Verification items for this drawing (mm, ordinates from the low corner). A direction names the side the tool comes from. Coordinates: 2 decimals unless noted, no trailing zeros. Order: outer loops, then holes, each group sorted by start corner. A loop starts at its lowest first (then second) coordinate and runs counter-clockwise, first axis right, second up. Notation, with made-up numbers: (33, -17) -> (70, -17) arc R22 cw to (70, 8) -> close; hole circle Ø11 at (61.5, 20.5). An arc over 180 degrees is marked (long way). Write item = value, one per line. Start each with the question number.
1. Cross-section at C-C on z = 12.7. Record the cut outline in (x, y).
2. Set-up check for the marked faces 4, 5, 6 and 7: record each of +Z, -Z, +X, -X, +Y, -Y from which the full face is reachable in a straight line by a thin tool's end or side.
3. Thickness scan on line 1 along Z through (x, y) = (18, 38.1); line 2 along Y through (x, z) = (19, 38.5); line 3 along Y through (x, z) = (23.5, 28.5). Record the ranges inside material, lowest first. Write a range as from..to.
4. Cross-section at A-A on y = 38.1. Record the cut outline in (x, z), plus the area to 3 significant figures.
5. Go/stop test with flat-tipped pins: P1, Ø12.5, axis at x = 11, y = 41, coming from the -Z side; P2, Ø12, axis at y = 8.5, z = 22, coming from the -X side; P3, Ø1, axis at x = 10, z = 43.5, coming from the -Y side. Record where each tip stops, or that it passes through.
6. Cross-section at D-D on x = 38.1. Record the cut outline in (y, z), plus the area to 3 significant figures.
7. Release check for a two-part mould opening along X. For the marked faces 1, 2 and 3 record: +X half, -X half, draft (parallel to the pull), parting line (faces both ways), or undercut.
8. Cross-section at B-B on x = 21. Record the cut outline in (y, z).
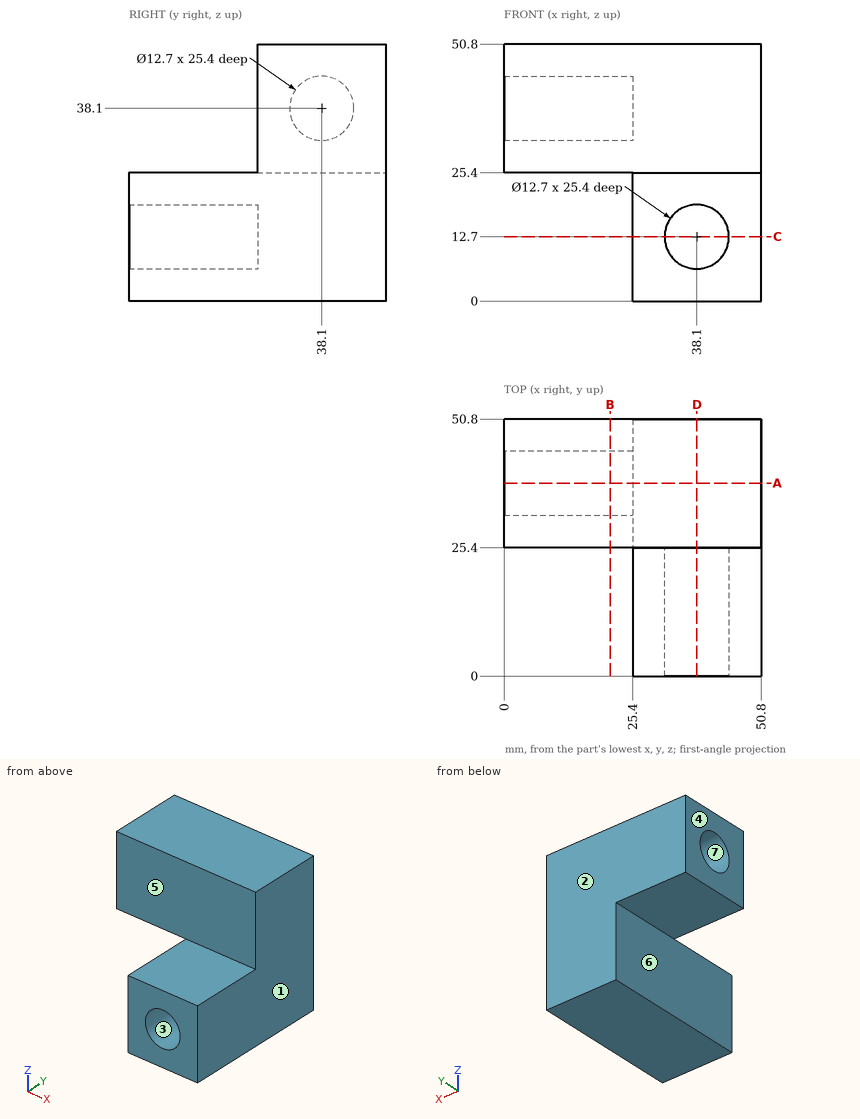
Worked out:
q1.outline = (25.4, 0) -> (31.75, 0) -> (31.75, 25.4) -> (44.45, 25.4) -> (44.45, 0) -> (50.8, 0) -> (50.8, 50.8) -> (25.4, 50.8) -> close
q2.face_4 = +Z, -Z, -X, +Y, -Y
q2.face_5 = +Z, +X, -X, -Y
q2.face_6 = -Z, -X, +Y, -Y
q2.face_7 = -X
q3.line_1 = 25.4..31.75, 44.45..50.8
q3.line_2 = 25.4..31.76, 44.44..50.8
q3.line_3 = 25.4..50.8
q4.outline = (0, 25.4) -> (25.4, 25.4) -> (25.4, 0) -> (50.8, 0) -> (50.8, 50.8) -> (0, 50.8) -> (0, 44.45) -> (25.4, 44.45) -> (25.4, 31.75) -> (0, 31.75) -> close
q4.area = 1,610 mm²
q5.P1 = 25.4
q5.P2 = 25.4
q5.P3 = 25.4
q6.outline = (0, 0) -> (50.8, 0) -> (50.8, 50.8) -> (25.4, 50.8) -> (25.4, 25.4) -> (0, 25.4) -> (0, 19.05) -> (25.4, 19.05) -> (25.4, 6.35) -> (0, 6.35) -> close
q6.area = 1,610 mm²
q7.face_1 = +X half
q7.face_2 = draft
q7.face_3 = undercut
q8.outline = (25.4, 25.4) -> (50.8, 25.4) -> (50.8, 50.8) -> (25.4, 50.8) -> close; hole circle Ø12.7 at (38.1, 38.1)
